Geometry check sheet. Reference: the model listing, model coordinates, mm. Face numbers are marked on the shaded views. A direction names the side the tool comes from. Coordinates: 2 decimals unless noted, no trailing zeros. Loops run counter-clockwise (first coordinate to the right, second up) from the corner with the lowest first, then second, coordinate; pieces in that order, holes last.
from build123d import *

# Parameters (mm, degrees)
SKETCH1_W           = 77
SKETCH1_H           = 50
SKETCH1_R           = 1.5
SKETCH1_W_2         = 32
SKETCH1_H_2         = 6.3
BOSS_EXTRUDE1_DEPTH = 2
BOSS_EXTRUDE2_DEPTH = 10
BOSS_EXTRUDE3_DEPTH = 2
CHAMFER1_SIZE       = 2
CUT_EXTRUDE1_REACH  = 97.131


with BuildPart() as part:
    # Sketch1 → Boss-Extrude1 (new body)
    with BuildSketch(Plane(origin=(0, 0, 0), x_dir=(1, 0, 0), z_dir=(0, 1, 0))):
        Rectangle(SKETCH1_W, SKETCH1_H)
        with Locations(Location((-36.25, 22.75, 0), (0, 0, 270))):
            Circle(SKETCH1_R, mode=Mode.SUBTRACT)
        with Locations(Location((36.25, 22.75, 0), (0, 0, 90))):
            Circle(SKETCH1_R, mode=Mode.SUBTRACT)
        with Locations(Location((36.25, -22.75, 0), (0, 0, 270))):
            Circle(SKETCH1_R, mode=Mode.SUBTRACT)
        with Locations(Location((-36.25, -22.75, 0), (0, 0, 90))):
            Circle(SKETCH1_R, mode=Mode.SUBTRACT)
        with Locations((10.75, 16.85)):
            Rectangle(SKETCH1_W_2, SKETCH1_H_2, mode=Mode.SUBTRACT)
        with Locations((10.75, -16.85)):
            Rectangle(SKETCH1_W_2, SKETCH1_H_2, mode=Mode.SUBTRACT)
    extrude(amount=BOSS_EXTRUDE1_DEPTH)

    # Sketch2 → Boss-Extrude2 (add)
    with BuildSketch(Plane(origin=(0, 2, 0), x_dir=(1, 0, 0), z_dir=(0, 1, 0))):
        Polygon((-38.5, 15), (-38.5, -15), (-5.25, -15), (-5.25, -13.7), (-5.25, -13), (-36.5, -13), (-36.5, 13), (-5.25, 13), (-5.25, 13.7), (-5.25, 15), align=None)
        Polygon((15.5, 13), (13.5, 13), (13.5, 9), (38.5, 9), (38.5, 11), (15.5, 11), align=None)
        Polygon((38.5, 11), (38.5, 9), (50.5, 9), (50.5, 6), (52.5, 6), (52.5, 11), align=None)
        Polygon((50.5, -9), (38.5, -9), (38.5, -11), (52.5, -11), (52.5, -6), (50.5, -6), align=None)
        Polygon((13.5, -9), (13.5, -13), (15.5, -13), (15.5, -11), (38.5, -11), (38.5, -9), align=None)
    extrude(amount=BOSS_EXTRUDE2_DEPTH)

    # Sketch3 → Boss-Extrude3 (add)
    with BuildSketch(Plane.XZ.offset(-2)):
        Polygon((38.5, 25), (52.5, 11), (52.5, -11), (38.5, -25), align=None)
    extrude(amount=BOSS_EXTRUDE3_DEPTH)

    # Chamfer1
    chamfer1_edges = [part.edges().sort_by_distance(p)[0] for p in [
        (-21.875, 2, -15),
        (34, 2, -11),
        (34, 2, 11),
        (-21.875, 2, 15),
    ]]
    chamfer(chamfer1_edges, length=CHAMFER1_SIZE)

    # Sketch4 → Cut-Extrude1 (cut, up to next)
    with BuildSketch(Plane.ZY.offset(38.5), mode=Mode.PRIVATE) as cut_extrude1_sk1:
        Polygon((-7.5, 6.556624327), (-7.5, 9.443375673), (-10, 10.886751346), (-12.5, 9.443375673), (-12.5, 6.556624327), (-10, 5.113248654), align=None)
    cut_extrude1_tool1 = extrude(cut_extrude1_sk1.sketch, amount=-CUT_EXTRUDE1_REACH, mode=Mode.PRIVATE) & part.part
    # Sketch4 → Cut-Extrude1 (cut, up to next)
    with BuildSketch(Plane.ZY.offset(38.5), mode=Mode.PRIVATE) as cut_extrude1_sk2:
        Polygon((0, 10.886751346), (0, 5.113248654), (2.5, 6.556624327), (2.5, 9.443375673), align=None)
    cut_extrude1_tool2 = extrude(cut_extrude1_sk2.sketch, amount=-CUT_EXTRUDE1_REACH, mode=Mode.PRIVATE) & part.part
    # Sketch4 → Cut-Extrude1 (cut, up to next)
    with BuildSketch(Plane.ZY.offset(38.5), mode=Mode.PRIVATE) as cut_extrude1_sk3:
        Polygon((-2.5, 6.556624327), (0, 5.113248654), (0, 10.886751346), (-2.5, 9.443375673), align=None)
    cut_extrude1_tool3 = extrude(cut_extrude1_sk3.sketch, amount=-CUT_EXTRUDE1_REACH, mode=Mode.PRIVATE) & part.part
    # Sketch4 → Cut-Extrude1 (cut, up to next)
    with BuildSketch(Plane.ZY.offset(38.5), mode=Mode.PRIVATE) as cut_extrude1_sk4:
        Polygon((12.5, 6.556624327), (12.5, 9.443375673), (10, 10.886751346), (7.5, 9.443375673), (7.5, 6.556624327), (10, 5.113248654), align=None)
    cut_extrude1_tool4 = extrude(cut_extrude1_sk4.sketch, amount=-CUT_EXTRUDE1_REACH, mode=Mode.PRIVATE) & part.part
    add(cut_extrude1_tool1.solids().sort_by_distance((-38.5, 8, -10))[0], mode=Mode.SUBTRACT)
    add(cut_extrude1_tool2.solids().sort_by_distance((-38.5, 8, 1.111111))[0], mode=Mode.SUBTRACT)
    add(cut_extrude1_tool3.solids().sort_by_distance((-38.5, 8, -1.111111))[0], mode=Mode.SUBTRACT)
    add(cut_extrude1_tool4.solids().sort_by_distance((-38.5, 8, 10))[0], mode=Mode.SUBTRACT)


solid = part.part
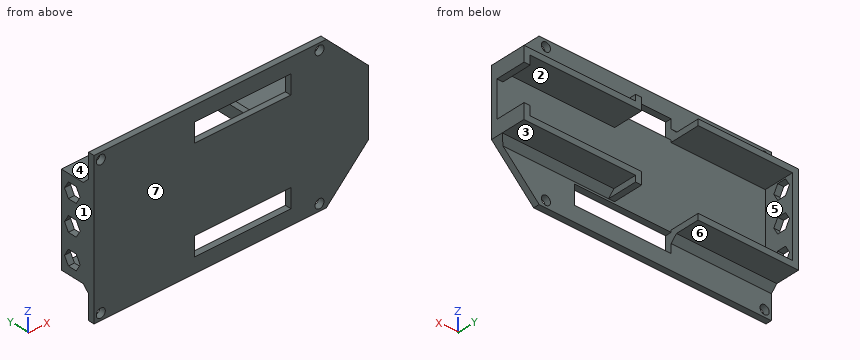
(1) Sectioned sample at C-C on z = -22.75. Record the cut outline in (x, y).
Findings:
outline: (-38.5, 0) - (-37.75, 0) - (-37.75, 2) - (-38.5, 2) - close; (-34.75, 0) - (34.75, 0) - (34.75, 2) - (-34.75, 2) - close; (37.75, 0) - (40.75, 0) - (40.75, 2) - (37.75, 2) - close
(2) Scan lines: L1, parallel to Z at x = 12, y = 1.5; L2, parallel to X at y = 1.4, z = -22.75; L3, parallel to X at y = 10.75, z = -8. Record each from-to range of solid material in increasing order.
Findings:
L1: z = -25 to -20, -13.7 to 13.7, 20 to 25
L2: x = -38.5 to -37.75, -34.75 to 34.75, 37.75 to 40.75
L3: x = -38.5 to -36.5, 50.5 to 52.5
(3) Sectioned sample at D-D on x = 36.25. Record the cut outline in (y, z), and give its area (3 significant figures).
Findings:
outline: (0, -25) - (2, -25) - (2, -24.25) - (0, -24.25) - close; (0, -21.25) - (2, -21.25) - (2, -13) - (4, -11) - (12, -11) - (12, -9) - (2, -9) - (2, 9) - (12, 9) - (12, 11) - (4, 11) - (2, 13) - (2, 21.25) - (0, 21.25) - close; (0, 24.25) - (2, 24.25) - (2, 25) - (0, 25) - close
area: 132 mm2
(4) Draft check along Z on the marked faces 4, 5, 6 and 7. Enter one of: +Z half, -Z half, draft (parallel to the pull), parting line (faces both ways), or undercut.
Findings:
face 4: +Z half
face 5: undercut
face 6: -Z half
face 7: draft
(5) Sectioned sample at A-A on x = -3.5. Record the cut outline in (y, z).
Findings:
outline: (0, -25) - (2, -25) - (2, -20) - (0, -20) - close; (0, -13.7) - (2, -13.7) - (2, 13.7) - (0, 13.7) - close; (0, 20) - (2, 20) - (2, 25) - (0, 25) - close
(6) Gauge pin test, flat ends, axial feed: pin 1 Ø0.6 at (x, y) = (-37, 8.5) entering from -Z; pin 2 Ø10 at (x, z) = (-1.5, -2) entering from +Y; pin 3 Ø1.6 at (x, y) = (51.5, 6) entering from +Z. Record the tip position at first contact, or that the pin passes through.
Findings:
pin 1: stops at z = -15
pin 2: stops at y = 2
pin 3: stops at z = 11
(7) Access from +Z, -Z, +X, -X, +Y, -Y to the whole of each face (thin tool, end or side, straight path). Record for the marked faces 1, 2 and 3.
Findings:
face 1: +Z, -Z, -X, +Y, -Y
face 2: +Y
face 3: -Z, +X, +Y
(8) Sectioned sample at B-B on z = -16. Record the cut outline in (x, y), and give its area (3 significant figures).
Findings:
outline: (-38.5, 0) - (-5.25, 0) - (-5.25, 3) - (-38.5, 3) - close; (26.75, 0) - (47.5, 0) - (47.5, 2) - (26.75, 2) - close
area: 141 mm2
